from build123d import *

# Parameters (mm, degrees)
F0_R     = 23
F1_DEPTH = 10
F2_R     = 22
F2_R_2   = 3
F2_R_3   = 2.15
F3_DEPTH = 7.5
F4_DEPTH = 2


with BuildPart() as f1:
    # F0 (on Top) → F1 (new body)
    with BuildSketch(Plane.XY):
        Circle(F0_R)
    extrude(amount=F1_DEPTH)

    # F2 (on face) → F3 (cut)
    with BuildSketch(Plane.XY.offset(10)):
        Circle(F2_R)
        Circle(F2_R_2, mode=Mode.SUBTRACT)
        Circle(F2_R_3)
    extrude(amount=-F3_DEPTH, mode=Mode.SUBTRACT)

    # F4 (cut): a face of the model
    f4_faces = [f1.faces().sort_by_distance(p)[0] for p in [
        (-2.9151471863, 0, 10),
    ]]
    extrude(f4_faces, amount=-F4_DEPTH, mode=Mode.SUBTRACT)


solid = f1.part
Input: part model. Units: mm. Frame: model coordinates. A direction names the side the tool comes from. Coordinates: 2 decimals unless noted, no trailing zeros. Loops run counter-clockwise (first coordinate to the right, second up) from the corner with the lowest first, then second, coordinate; pieces in that order, holes last.
(1) Set-up query: faces 4 (the face through (-2.15, 0.09, 5.29)), 5 (the face through (12, -19, 10)). Return all of +Z, -Z, +X, -X, +Y, -Y with unobstructed straight access to the full face (end or side cutting, diameter ignored); none if empty.
(2) Pull-direction query (X, two-part tool) for faces 1 (the face through (0, -5, 2.5)), 2 (the face through (0, 0, 0)), 3 (the face through (-2.994, 22.804, 4.93)); classes: released by +X, released by -X, zero draft, split by the parting line, or undercut.
(3) Section B-B on y = -14.5. Return the cut outline in (x, z), then the cut area to 3 significant figures.
(4) Section A-A on z = 7. Return the cut outline in (x, y), then the cut area to 3 significant figures.
(5) Material intervals for probe 1 along Y at (x, z) = (0, 5); probe 2 along Z at (x, y) = (7, 12); probe 3 along Y at (x, z) = (-11.5, 5.75) (3 decimals), sorted ascending.
(6) First-contact query: pin 1 Ø4 at (y, z) = (13, 7.5) entering from -X; pin 2 Ø1.5 at (x, y) = (16, 9) entering from +Z; pin 3 Ø2 at (x, y) = (-1, 1) entering from +Z. Flat tips, straight axial feed; report the tip coordinate or a pass-through.
(7) Section C-C on x = 0. Return the cut outline in (y, z), then the cut area to 3 significant figures.
Data:
1. face 4: +Z
1. face 5: +Z, +X, -X, +Y, -Y
2. face 1: undercut
2. face 2: zero draft
2. face 3: split by the parting line
3. outline: (-17.85, 0) - (17.85, 0) - (17.85, 10) - (16.55, 10) - (16.55, 2.5) - (-16.55, 2.5) - (-16.55, 10) - (-17.85, 10) - close
3. area: 109 mm2
4. outline: circle Ø46 at (0, 0); circle Ø6 at (0, 0); hole circle Ø44 at (0, 0); hole circle Ø4.3 at (0, 0)
4. area: 155 mm2
5. probe 1: y = -23 to -22, -3 to -2.15, 2.15 to 3, 22 to 23
5. probe 2: z = 0 to 2.5
5. probe 3: y = -19.919 to -18.755, 18.755 to 19.919
6. pin 1: stops at x = -20.2
6. pin 2: stops at z = 2.5
6. pin 3: stops at z = 8
7. outline: (-23, 0) - (23, 0) - (23, 10) - (22, 10) - (22, 2.5) - (3, 2.5) - (3, 8) - (2.15, 8) - (2.15, 2.5) - (-2.15, 2.5) - (-2.15, 8) - (-3, 8) - (-3, 2.5) - (-22, 2.5) - (-22, 10) - (-23, 10) - close
7. area: 139 mm2
